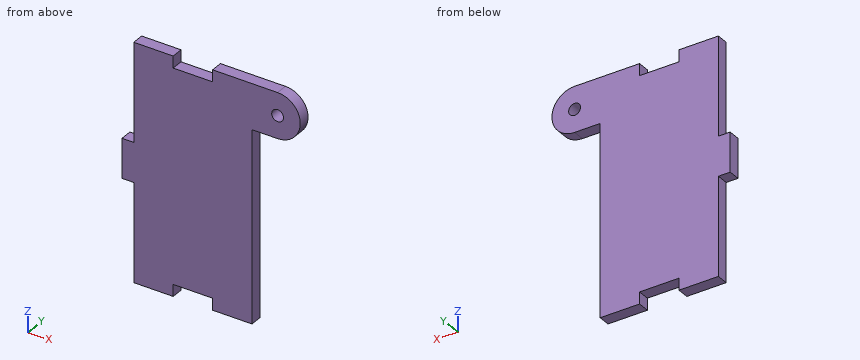
from build123d import *

# Parameters (mm, degrees)
SKETCH1_R           = 1.5
BOSS_EXTRUDE1_DEPTH = 3


with BuildPart() as part:
    # Sketch1 → Boss-Extrude1 (new body)
    with BuildSketch(Plane(origin=(0, 0, 0), x_dir=(1, 0, 0), z_dir=(0, 1, 0))):
        with BuildLine():
            Line((21.5, -18.5), (15, -18.5))
            Line((15, -18.5), (15, -5))
            Line((15, -5), (15, 30))
            Line((15, 30), (5, 30))
            Line((5, 30), (5, 27))
            Line((5, 27), (-5, 27))
            Line((-5, 27), (-5, 30))
            Line((-5, 30), (-15, 30))
            Line((-15, 30), (-15, 5))
            Line((-15, 5), (-18, 5))
            Line((-18, 5), (-18, -5))
            Line((-18, -5), (-15, -5))
            Line((-15, -5), (-15, -30))
            Line((-15, -30), (-5, -30))
            Line((-5, -30), (-5, -27))
            Line((-5, -27), (5, -27))
            Line((5, -27), (5, -30))
            Line((5, -30), (15, -30))
            Line((15, -30), (21.5, -30))
            ThreePointArc((21.5, -30), (27.25, -24.25), (21.5, -18.5))
        make_face()
        with Locations(Location((21.5, -24.25, 0), (0, 0, 270))):
            Circle(SKETCH1_R, mode=Mode.SUBTRACT)
    extrude(amount=BOSS_EXTRUDE1_DEPTH)


solid = part.part
Geometry check sheet. Reference: the model listing, model coordinates, mm. Give positions to 0.01 mm unless a question says otherwise; leave off trailing zeros. Loops run counter-clockwise (first coordinate to the right, second up) from the corner with the lowest first, then second, coordinate; pieces in that order, holes last.
(1) Section check A-A on z = 24.25. Record the cut outline in (x, y), then the cut area to 3 significant figures.
From the geometry:
outline: (-15, 0) - (20, 0) - (20, 3) - (-15, 3) - close; (23, 0) - (27.25, 0) - (27.25, 3) - (23, 3) - close
area: 118 mm2
(2) Depth check by flat-ended pin: pin 1 Ø1.5 at (x, y) = (-16, 1) entering from +Z; pin 2 Ø1.5 at (y, z) = (1.5, 3) entering from +X; pin 3 Ø12 at (x, z) = (-2, -4.5) entering from -Y; pin 4 Ø1.8 at (x, z) = (21.5, 24.25) entering from +Y. Enter the tip coordinate at first touch or a pass-through.
From the geometry:
pin 1: stops at z = 5
pin 2: stops at x = 15
pin 3: stops at y = 0
pin 4: passes through
(3) Section check D-D on z = -13.5. Record the cut outline in (x, y), then the cut area to 3 significant figures.
From the geometry:
outline: (-15, 0) - (15, 0) - (15, 3) - (-15, 3) - close
area: 90.0 mm2
(4) Thickness scan on L1, parallel to X at y = 2.2, z = 24.25; L2, parallel to X at y = 1.9, z = -8; L3, parallel to X at y = 1.55, z = 4. Record the ranges inside material, lowest first.
From the geometry:
L1: x = -15 to 20, 23 to 27.25
L2: x = -15 to 15
L3: x = -18 to 15
(5) Section check C-C on x = 18.5. Record the cut outline in (y, z), then the cut area to 3 significant figures.
From the geometry:
outline: (0, 18.5) - (3, 18.5) - (3, 30) - (0, 30) - close
area: 34.5 mm2
(6) Section check B-B on y = 1.3. Record the cut outline in (x, z).
From the geometry:
outline: (-18, -5) - (-15, -5) - (-15, -30) - (-5, -30) - (-5, -27) - (5, -27) - (5, -30) - (15, -30) - (15, 18.5) - (21.5, 18.5) arc R5.75 ccw to (21.5, 30) - (5, 30) - (5, 27) - (-5, 27) - (-5, 30) - (-15, 30) - (-15, 5) - (-18, 5) - close; hole circle Ø3 at (21.5, 24.25)
